Here's how the part is built. I have some questions about the finished solid (model axes, mm). Face numbers are marked on the shaded views. A direction names the side the tool comes from. Give positions to 0.01 mm unless a question says otherwise; leave off trailing zeros. Write each loop counter-clockwise with the first axis right and the second up, starting at its lowest first coordinate (ties: lowest second). Pieces come first, ordered by that corner, then holes. Notation, with made-up numbers: (2.5, -9.75) -> (31.5, -9.75) arc R16 cw to (31.5, 10.25) -> close; hole circle Ø7 at (-39.5, -37.75). An arc over 180 degrees is marked (long way). Return JSON: item names as keys, results as strings.
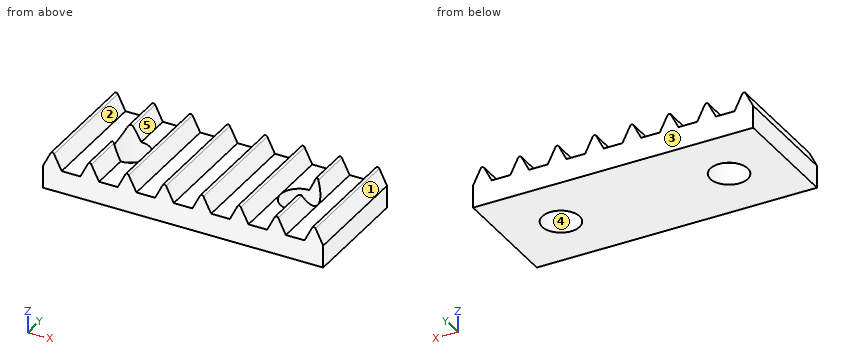
Autodesk Inventor part; units mm, degrees
ref_plane "YZ Plane" through (0, 0, 0) normal (1, 0, 0) x (0, 1, 0)
ref_plane "XZ Plane" through (0, 0, 0) normal (0, 1, 0) x (-1, 0, 0)
ref_plane "XY Plane" through (0, 0, 0) normal (0, 0, 1) x (1, 0, 0)
sketch "Sketch1" plane through (0, 0, 0) normal (0, 0, 1) x (1, 0, 0)
  line L0 (0, 0) -> (0, 6.2)
  line L1 (0, 6.2) -> (15, 6.2)
  line L2 (15, 6.2) -> (15, 0)
  line L3 (15, 0) -> (0, 0)
  dimension "d0" = 6.2
  dimension "d1" = 15
extrude "Extrusion1" add sketch "Sketch1" along normal blind 1.2
sketch "Sketch2" plane through (0, 0, 0) normal (0, -1, 0) x (1, 0, 0)
  line L0 (0, 0) -> (0, 1.2)
  line L1 (0, 1.2) -> (0.5, 1.2)
  line L2 (15, 1.2) -> (0, 1.2)
  line L3 (0.5, 1.2) -> (0.5, 2.2)
  line L4 (0.5, 2.2) -> (0, 1.2)
  line L5 (0.5, 1.2) -> (1, 1.2)
  line L6 (1, 1.2) -> (0.5, 2.2)
  dimension "d4" = 0.5
  dimension "d5" = 1
  dimension "d6" = 0.5
extrude "Extrusion2" add sketch "Sketch2" against normal blind 6.2
fillet "Fillet1" radius 0.1 1 edges at (0.5, 3.1, 2.2)
pattern_linear "Rectangular Pattern1" count 8 spacing 2 along (1, 0, 0) of "Fillet1", "Extrusion2"
sketch "Sketch3" plane through (0, 0, 0) normal (0, 0, -1) x (-1, 0, 0)
  circle A0 centre (-3, 3.1) radius 1
  circle A1 centre (-12, 3.1) radius 1
  line L0 (0, 6.2) -> (0, 0)
  line L1 (-15, 0) -> (-15, 6.2)
  dimension "d13" = 2
  dimension "d14" = 2
  dimension "d15" = 3
  dimension "d16" = 3
extrude "Extrusion3" cut sketch "Sketch3" against normal blind 6.2
properties part number "time belt coupling"
1. Suppose I cut it at C-C, the plane x = 13.75. List the corners of the cut face in (y, z) for me, and give its area (3 significant figures).
Taken from the geometry:
{"outline": "(0, 0) -> (6.2, 0) -> (6.2, 1.2) -> (0, 1.2) -> close", "area": "7.44 mm²"}
2. For pin 1 Ø1.1 at (x, y) = (1.5, 2.5) entering from +Z; pin 2 Ø0.8 at (x, y) = (13.5, 4.5) entering from +Z, each with a flat end and sliding along its axis, tell me the tip position at first contact or that it passes through.
Taken from the geometry:
{"pin 1": "stops at z = 1.3", "pin 2": "stops at z = 1.2"}
3. If I drill on line 1 (X direction, y = 3.1, z = 1.05); line 2 (Y direction, x = 3, z = 1.15); line 3 (X direction, y = 3.5, z = 0.25), over which ranges is the centre line in solid material (lowest first)? Write a range as [from, to].
Taken from the geometry:
{"line 1": "x = [0, 2], [4, 11], [13, 15]", "line 2": "y = [0, 2.1], [4.1, 6.2]", "line 3": "x = [0, 2.08], [3.92, 11.08], [12.92, 15]"}
4. Which directions (+Z, -Z, +X, -X, +Y, -Y) give clear straight access to the entire face, cutting with the end or side of a thin tool? Please do the marked faces 1 and 2.
Taken from the geometry:
{"face 1": "+Z, +X, +Y, -Y", "face 2": "+Z, +Y, -Y"}
5. If we mould it in two halves opening along Y, with no side actions, what happens to the marked faces 3, 4 and 5? For each: released by +Y, released by -Y, zero draft, split by the parting line, or undercut.
Taken from the geometry:
{"face 3": "released by +Y", "face 4": "undercut", "face 5": "zero draft"}
6. Suppose I cut it at A-A, the plane z = 1.05. List the corners of the cut face in (x, y) for me, and give its area (3 significant figures).
Taken from the geometry:
{"outline": "(0, 0) -> (15, 0) -> (15, 6.2) -> (0, 6.2) -> close; hole circle Ø2 at (3, 3.1); hole circle Ø2 at (12, 3.1)", "area": "86.7 mm²"}
